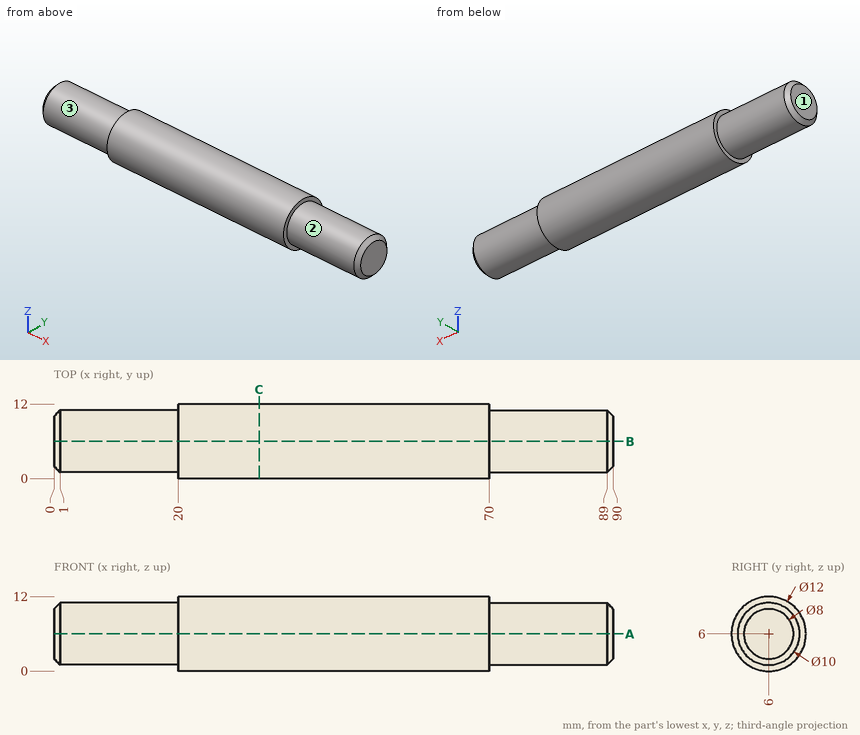
Print and shaded views of the part. All mm, measured from the part's lowest x, y and z. A direction names the side the tool comes from. Coordinates: 2 decimals unless noted, no trailing zeros. Write each loop counter-clockwise with the first axis right and the second up, starting at its lowest first coordinate (ties: lowest second). Pieces come first, ordered by that corner, then holes.
(1) 3-axis set-ups, long thin cutter, end or side, ignore diameter. For the marked faces 1, 2 and 3: which of +Z, -Z, +X, -X, +Y, -Y reach the whole face in a straight line?
(2) Cut at A-A, the plane z = 6. List the corners of the cut face in (x, y), and give its area (3 significant figures).
(3) Flat gauge pins, fed straight in: pin 1 (6 mm diameter, centred on y = 1, z = 4.5, fed in from -X); pin 2 (1 mm diameter, centred on x = 14, z = 5.5, fed in from +Y); pin 3 (1.5 mm diameter, centred on x = 22.5, y = 8.5, fed in from -Z). Where does each tip first touch, or does it go through?
(4) Drill centre lines: probe 1 along X at (y, z) = (7.25, 11.25); probe 2 along Y at (x, z) = (84.5, 6.25); probe 3 along Z at (x, y) = (31, 5.75). Where is each one in solid material? Low to high.
(5) Cut at C-C, the plane x = 33. List the corners of the cut face in (y, z).
Geometry says:
1. face 1: +Z, -Z, -X, +Y, -Y
1. face 2: +X
1. face 3: -X
2. outline: (0, 2) - (1, 1) - (20, 1) - (20, 0) - (70, 0) - (70, 1) - (89, 1) - (90, 2) - (90, 10) - (89, 11) - (70, 11) - (70, 12) - (20, 12) - (20, 11) - (1, 11) - (0, 10) - close
2. area: 998 mm2
3. pin 1: stops at x = 0
3. pin 2: stops at y = 11
3. pin 3: stops at z = 0.26
4. probe 1: x = 20 to 70
4. probe 2: y = 1.01 to 10.99
4. probe 3: z = 0.01 to 11.99
5. outline: circle Ø12 at (6, 6)
